```python
from build123d import *

# Parameters (mm, degrees)
SZKIC1_R                    = 3.3
SZKIC1_R_2                  = 11
DODANIE_WYCI_GNI_CIE2_DEPTH = 15
SZKIC2_W                    = 17
SZKIC2_H                    = 8
SZKIC2_H_2                  = 8.035759956
WYTNIJ_WYCI_GNI_CIE1_DEPTH  = 16
SZKIC3_R                    = 6
WYTNIJ_WYCI_GNI_CIE2_DEPTH  = 45


with BuildPart() as part:
    # Szkic1 → Dodanie-wyciągnięcie2 (new body)
    with BuildSketch(Plane.XY):
        with BuildLine():
            Line((-18.894443628, 22), (18.894443628, 22))
            ThreePointArc((18.894443628, 22), (29, 0), (18.894443628, -22))
            Line((18.894443628, -22), (-18.894443628, -22))
            ThreePointArc((-18.894443628, -22), (-29, 0), (-18.894443628, 22))
        make_face()
        with Locations((-23.5, 0)):
            Circle(SZKIC1_R, mode=Mode.SUBTRACT)
        with Locations((-16.617009358, 16.617009358)):
            Circle(SZKIC1_R, mode=Mode.SUBTRACT)
        with Locations((16.617009358, 16.617009358)):
            Circle(SZKIC1_R, mode=Mode.SUBTRACT)
        with Locations((23.5, 0)):
            Circle(SZKIC1_R, mode=Mode.SUBTRACT)
        with Locations((16.617009358, -16.617009358)):
            Circle(SZKIC1_R, mode=Mode.SUBTRACT)
        with Locations((-16.617009358, -16.617009358)):
            Circle(SZKIC1_R, mode=Mode.SUBTRACT)
        Circle(SZKIC1_R_2, mode=Mode.SUBTRACT)
    extrude(amount=DODANIE_WYCI_GNI_CIE2_DEPTH)

    # Szkic2 → Wytnij-wyciągnięcie1 (cut, through all)
    with BuildSketch(Plane.XY.offset(15)):
        with Locations((0, -11)):
            Rectangle(SZKIC2_W, SZKIC2_H)
        with Locations((0, 11)):
            Rectangle(SZKIC2_W, SZKIC2_H_2)
    extrude(amount=-WYTNIJ_WYCI_GNI_CIE1_DEPTH, mode=Mode.SUBTRACT)

    # Szkic3 → Wytnij-wyciągnięcie2 (cut, through all)
    with BuildSketch(Plane.XZ.offset(22)):
        with Locations((0, 15)):
            Circle(SZKIC3_R)
    extrude(amount=-WYTNIJ_WYCI_GNI_CIE2_DEPTH, mode=Mode.SUBTRACT)


solid = part.part
```
Source: CAD feature listing. Evaluate the final solid. Frame: model axes, mm. A direction names the side the tool comes from. Round coordinates to 2 decimals unless told otherwise and drop trailing zeros. Loops run counter-clockwise (first coordinate to the right, second up) from the corner with the lowest first, then second, coordinate; pieces in that order, holes last. Notation, with made-up numbers: M 80,16.25 L 110,16.25 A17 cw 110,30.25 Z; hole C 24.25,9.5 d8. An arc over 180 degrees is marked long. Put each result on its own line as item: value.
(1) First-contact query: pin 1 (5.5 mm diameter, centred on x = -23.5, y = 0, fed in from -Z); pin 2 (4 mm diameter, centred on y = 10.5, z = 11, fed in from -X); pin 3 (1.5 mm diameter, centred on y = 17, z = 3, fed in from +X); pin 4 (9 mm diameter, centred on y = -12, z = 4, fed in from +X). Flat tips, straight axial feed; report the tip coordinate or a pass-through.
Solutions:
pin 1: through
pin 2: x = -27.73
pin 3: x = 24.02
pin 4: x = 28.01
(2) Section D-D, the plane z = 1.75. State how many separate pieces and enclosed holes the cut face has, and give its area (3 significant figures).
Solutions:
separate pieces: 1
enclosed holes: 7
area: 1,520 mm²
(3) Pull-direction query (Y, two-part tool) for faces 3 (the face through (8.5, -11, 8)), 4 (the face through (0, -22, 7)), 5 (the face through (0, 22, 7)); classes: released by +Y, released by -Y, zero draft, split by the parting line, or undercut.
Solutions:
face 3: undercut
face 4: released by -Y
face 5: released by +Y
(4) Section A-A, the plane y = 0. Return loops of the section in (x, z).
Solutions:
outline: M -29,0 L -26.8,0 L -26.8,15 L -29,15 Z; M -20.2,0 L -11,0 L -11,15 L -20.2,15 Z; M 11,0 L 20.2,0 L 20.2,15 L 11,15 Z; M 26.8,0 L 29,0 L 29,15 L 26.8,15 Z
(5) Ray query, line 1 (X direction, y = 19.5, z = 14.25); line 2 (Y direction, x = -0.5, z = 1); line 3 (Y direction, x = 18.5, z = 12). Return the intervals inside material, ascending. Write a range as [from, to].
Solutions:
line 1: [-21.47, -18.22], [-15.01, -5.95], [5.95, 15.01], [18.22, 21.47]
line 2: [-22, -15], [15.02, 22]
line 3: [-22, -19.33], [-13.91, 13.91], [19.33, 22]
(6) Section B-B, the plane x = 0. Return loops of the section in (y, z), and give its area (3 significant figures).
Solutions:
outline: M -22,0 L -15,0 L -15,9 L -22,9 Z; M 15.02,0 L 22,0 L 22,9 L 15.02,9 Z
area: 126 mm²
(7) Section C-C, the plane x = -16. Return loops of the section in (y, z).
Solutions:
outline: M -22,0 L -19.86,0 L -19.86,15 L -22,15 Z; M -13.38,0 L 13.38,0 L 13.38,15 L -13.38,15 Z; M 19.86,0 L 22,0 L 22,15 L 19.86,15 Z
(8) Access query for faces 1 (the face through (0, 18, 9)), 2 (the face through (-8.5, 11, 8)). Directions: +Z, -Z, +X, -X, +Y, -Y. A direction counts if a zero-diameter tool reaches every point of the face in a straight line with its end or side. Return the directions, or none.
Solutions:
face 1: +Z, +Y, -Y
face 2: +Z, -Z
